Geometry: final body of the model. Coordinates: model frame, mm. A direction names the side the tool comes from. Give positions to 0.01 mm unless a question says otherwise; leave off trailing zeros. Loops run counter-clockwise (first coordinate to the right, second up) from the corner with the lowest first, then second, coordinate; pieces in that order, holes last.
```python
from build123d import *

# Parameters (mm, degrees)
CUT_EXTRUDE2_DEPTH = 2.5
CUT_EXTRUDE3_DEPTH = 2.5
FILLET1_R          = 1
FILLET2_R          = 1


with BuildPart() as part:
    # Sketch1 → Revolve1 (revolve)
    with BuildSketch(Plane.XY, mode=Mode.PRIVATE) as revolve1_sk:
        Polygon((16.777055999, 0), (16.777055999, 12.5), (50.777055999, 12.5), (50.777055999, 13), (117.777055999, 13), (117.777055999, 12.5), (211.777055999, 12.5), (211.777055999, 0), align=None)
    revolve(revolve1_sk.sketch.rotate(Axis((0, 0, 0), (1, 0, 0)), 180), axis=Axis((0, 0, 0), (1, 0, 0)))

    # Sketch2 → Cut-Extrude2 (cut)
    with BuildSketch(Plane.XY.offset(12.5)):
        with BuildLine():
            Line((120.977055999, 2.5), (143.977055999, 2.5))
            ThreePointArc((143.977055999, 2.5), (146.477055999, 0), (143.977055999, -2.5))
            Line((143.977055999, -2.5), (120.977055999, -2.5))
            ThreePointArc((120.977055999, -2.5), (118.477055999, 0), (120.977055999, 2.5))
        make_face()
    extrude(amount=-CUT_EXTRUDE2_DEPTH, mode=Mode.SUBTRACT)

    # Sketch3 → Cut-Extrude3 (cut)
    with BuildSketch(Plane.XY.offset(13)):
        with BuildLine():
            Line((68.277055999, 2.5), (91.277055999, 2.5))
            ThreePointArc((91.277055999, 2.5), (93.777055999, 0), (91.277055999, -2.5))
            Line((91.277055999, -2.5), (68.277055999, -2.5))
            ThreePointArc((68.277055999, -2.5), (65.777055999, 0), (68.277055999, 2.5))
        make_face()
    extrude(amount=-CUT_EXTRUDE3_DEPTH, mode=Mode.SUBTRACT)

    # Fillet1
    fillet1_edges = [part.edges().sort_by_distance(p)[0] for p in [
        (211.777055999, 12.5, 0),
    ]]
    fillet(fillet1_edges, radius=FILLET1_R)

    # Fillet2
    fillet2_edges = [part.edges().sort_by_distance(p)[0] for p in [
        (16.777055999, 12.5, 0),
    ]]
    fillet(fillet2_edges, radius=FILLET2_R)


solid = part.part
```
Q1. Section query C-C, the plane x = 128.5. Return loops of the section in (y, z).
Q2. Section query A-A, the plane y = 0. Return loops of the section in (x, z).
Q3. Pin query (flat end, axial travel): pin 1 Ø0.7 at (x, z) = (79, 11.5) entering from +Y; pin 2 Ø1.1 at (x, z) = (132, 11) entering from +Y; pin 3 Ø5.5 at (x, y) = (126, -0.5) entering from +Z. Return the tip coordinate at first contact, or that it passes through.
Q4. Section query D-D, the plane x = 38.5. Return loops of the section in (y, z).
Q5. Material intervals for probe 1 along Y at (x, z) = (55.5, -0.5); probe 2 along X at (y, z) = (11.5, -2.5); probe 3 along Z at (x, y) = (184, -0.25), sorted ascending.
Q6. Section query B-B, the plane z = 0. Return loops of the section in (x, y).
Q7. Mould query, pull axis X, two halves, no side actions, for faces 1 (the face through (211.777, 0, 0)), 2 (the face through (16.777, 0, 0)), 3 (the face through (133, 0, 10)). Classes: +X half, -X half, draft (parallel to the pull), parting line (faces both ways), or undercut.
Q8. Reachability of faces 4 (the face through (80, 0, 10.5)), 5 (the face through (164.928, -11.923, -3.755)), 6 (the face through (34.508, -11.923, -3.755)) from +Z, -Z, +X, -X, +Y, -Y: full face, straight path, thin tool, end or side. Return the list, or none.
Resolved:
1. outline: (-2.5, 10) - (-2.5, 12.25) arc R12.5 ccw (long way) to (2.5, 12.25) - (2.5, 10) - close
2. outline: (16.78, -11.5) arc R1 ccw to (17.78, -12.5) - (50.78, -12.5) - (50.78, -13) - (117.78, -13) - (117.78, -12.5) - (210.78, -12.5) arc R1 ccw to (211.78, -11.5) - (211.78, 11.5) arc R1 ccw to (210.78, 12.5) - (146.48, 12.5) - (146.48, 10) - (118.48, 10) - (118.48, 12.5) - (117.78, 12.5) - (117.78, 13) - (93.78, 13) - (93.78, 10.5) - (65.78, 10.5) - (65.78, 13) - (50.78, 13) - (50.78, 12.5) - (17.78, 12.5) arc R1 ccw to (16.78, 11.5) - close
3. pin 1: stops at y = 6.68
3. pin 2: stops at y = 6.86
3. pin 3: stops at z = 12.25
4. outline: circle Ø25 at (0, 0)
5. probe 1: y = -12.99 to 12.99
5. probe 2: x = 16.81 to 211.74
5. probe 3: z = -12.5 to 12.5
6. outline: (16.78, -11.5) arc R1 ccw to (17.78, -12.5) - (50.78, -12.5) - (50.78, -13) - (117.78, -13) - (117.78, -12.5) - (210.78, -12.5) arc R1 ccw to (211.78, -11.5) - (211.78, 11.5) arc R1 ccw to (210.78, 12.5) - (117.78, 12.5) - (117.78, 13) - (50.78, 13) - (50.78, 12.5) - (17.78, 12.5) arc R1 ccw to (16.78, 11.5) - close
7. face 1: +X half
7. face 2: -X half
7. face 3: undercut
8. face 4: +Z
8. face 5: +X
8. face 6: -X
